Verification items for the finished model (mm, model axes). Face numbers are marked on the shaded views. Give positions to 0.01 mm unless a question says otherwise; leave off trailing zeros. Order: outer loops, then holes, each group sorted by start corner. A loop starts at its lowest first (then second) coordinate and runs counter-clockwise, first axis right, second up.
(1) Mould release check, pull along X, two halves, no side actions. Record for the marked faces 1 and 2: pulls with the +X half, pulls with the -X half, needs draft (parallel to the pull), parting line crosses it, or undercut.
(2) Sectioned sample at A-A on z = 5. Record the cut outline in (x, y) (3 decimals).
(3) Sectioned sample at C-C on x = 0. Record the cut outline in (y, z) (3 decimals), plus the area to 3 significant figures.
(4) Sectioned sample at D-D on y = -19.5. Record the cut outline in (x, z), plus the area to 3 significant figures.
(5) Sectioned sample at B-B on y = -70. Record the cut outline in (x, z), plus the area to 3 significant figures.
(6) Scan lines: L1, parallel to X at y = -66.5, z = 5.5; L2, parallel to Z at x = 0.5, y = -37; L3, parallel to Z at x = 8.5, y = -73. Record each from-to range of solid material in increasing order.
(7) Gauge pin test, flat ends, axial feed: pin 1 (8 mm diameter, centred on x = -3.5, y = -22, fed in from +Z); pin 2 (0.6 mm diameter, centred on y = -61, z = 5.5, fed in from -X); pin 3 (1.5 mm diameter, centred on x = 3, y = -68, fed in from +Z); pin 4 (4.5 mm diameter, centred on x = -10.5, y = -70, fed in from -Z). Record the tip position at first contact, or that the pin passes through.
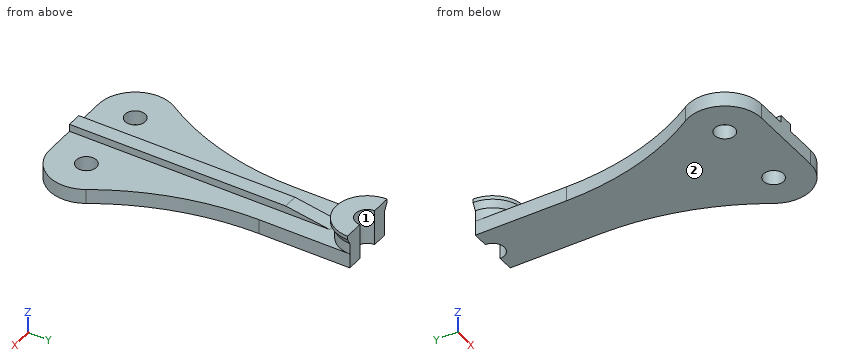
```python
from build123d import *

# Parameters (mm, degrees)
SKETCH1_R           = 2.75
BOSS_EXTRUDE1_DEPTH = 4
REVOLVE1_ANGLE      = 180
BOSS_EXTRUDE2_DEPTH = 2
BOSS_EXTRUDE3_DEPTH = 4


with BuildPart() as part:
    # Sketch1 → Boss-Extrude1 (new body)
    with BuildSketch(Plane.XY):
        with BuildLine():
            Line((-10.5, -60), (-7.5, -60))
            Line((-7.5, -60), (-7.5, 0))
            Line((-7.5, 0), (-3.175, 0))
            ThreePointArc((-3.175, 0), (0, -3.175), (3.175, 0))
            Line((3.175, 0), (7.5, 0))
            Line((7.5, 0), (7.5, -60))
            Line((7.5, -60), (10.5, -60))
            ThreePointArc((10.5, -60), (20.5, -70), (10.5, -80))
            Line((10.5, -80), (-10.5, -80))
            ThreePointArc((-10.5, -80), (-20.5, -70), (-10.5, -60))
        make_face()
        with Locations((-10.5, -70)):
            Circle(SKETCH1_R, mode=Mode.SUBTRACT)
        with Locations((10.5, -70)):
            Circle(SKETCH1_R, mode=Mode.SUBTRACT)
    extrude(amount=BOSS_EXTRUDE1_DEPTH)

    # Sketch2 → Revolve1 (revolve)
    with BuildSketch(Plane(origin=(0, 0, 0), x_dir=(1, 0, 0), z_dir=(0, 1, 0))):
        Polygon((7.5, -4), (3.175, -4), (3.175, -9.732050808), (8.5, -9.732050808), (8.5, -8.732050808), (7.5, -7), align=None)
    revolve(axis=Axis((0, 0, 0), (0, 0, -1)), revolution_arc=REVOLVE1_ANGLE)

    # Sketch3 → Boss-Extrude2 (add, symmetric)
    with BuildSketch(Plane(origin=(0, 0, 0), x_dir=(0, 0, -1), z_dir=(1, 0, 0))):
        Polygon((-4, -9), (-6, -21), (-6, -80), (-4, -80), align=None)
    extrude(amount=BOSS_EXTRUDE2_DEPTH, both=True)

    # Sketch4 → Boss-Extrude3 (add)
    with BuildSketch(Plane.XY.offset(4)):
        with BuildLine():
            Line((-7.5, -60), (-10.5, -60))
            ThreePointArc((-10.5, -60), (-15.339942392, -61.249288164), (-18.970588235, -64.685008471))
            ThreePointArc((-18.970588235, -64.685008471), (-10.424671758, -45.562558961), (-7.5, -24.822572008))
            Line((-7.5, -24.822572008), (-7.5, -60))
        make_face()
        with BuildLine():
            Line((7.5, -60), (7.5, -24.822572008))
            ThreePointArc((7.5, -24.822572008), (10.424671758, -45.562558961), (18.970588235, -64.685008471))
            ThreePointArc((18.970588235, -64.685008471), (15.339942392, -61.249288164), (10.5, -60))
            Line((10.5, -60), (7.5, -60))
        make_face()
    extrude(amount=-BOSS_EXTRUDE3_DEPTH)


solid = part.part
```
Ans:
1. face 1: undercut
1. face 2: needs draft
2. outline: (-7.5, 0) arc R7.5 ccw to (7.5, 0) - (3.175, 0) arc R3.175 cw to (-3.175, 0) - close; (-2, -80) - (2, -80) - (2, -15) - (-2, -15) - close
3. outline: (-80, 0) - (-3.175, 0) - (-3.175, 9.732) - (-8.5, 9.732) - (-8.5, 8.732) - (-7.5, 7) - (-7.5, 4) - (-9, 4) - (-21, 6) - (-80, 6) - close
3. area: 464 mm2
4. outline: (-7.5, 0) - (7.5, 0) - (7.5, 4) - (2, 4) - (2, 5.75) - (-2, 5.75) - (-2, 4) - (-7.5, 4) - close
4. area: 67.0 mm2
5. outline: (-20.5, 0) - (-13.25, 0) - (-13.25, 4) - (-20.5, 4) - close; (-7.75, 0) - (7.75, 0) - (7.75, 4) - (2, 4) - (2, 6) - (-2, 6) - (-2, 4) - (-7.75, 4) - close; (13.25, 0) - (20.5, 0) - (20.5, 4) - (13.25, 4) - close
5. area: 128 mm2
6. L1: x = -2 to 2
6. L2: z = 0 to 6
6. L3: z = 0 to 4
7. pin 1: stops at z = 6
7. pin 2: stops at x = -2
7. pin 3: stops at z = 4
7. pin 4: passes through
